Can you work these out from the model? Positions are in its coordinate system, mm. A direction names the side the tool comes from. Give positions to 0.01 mm unless a question says otherwise; leave off trailing zeros. Loops run counter-clockwise (first coordinate to the right, second up) from the corner with the lowest first, then second, coordinate; pieces in that order, holes last. Notation, with made-up numbers: M 38.5,-24.75 L 59.5,-24.75 A31 ccw 59.5,9.25 Z; hole C -8.75,69.5 d7. An arc over 180 degrees is marked long. Answer as a JSON object with one key per item and string values.
Autodesk Fusion 360 part; units mm, degrees
sketch "Sketch1" plane through (0, 0, 0) normal (0, 1, 0) x (1, 0, 0)
  line L0 (32.8, 42.5) -> (-32.8, 42.5)
  line L1 (-32.8, 42.5) -> (-32.8, -42.5)
  line L2 (-32.8, -42.5) -> (32.8, -42.5)
  line L3 (32.8, -42.5) -> (32.8, 42.5)
  line L4 (32.8, 42.5) -> (-32.8, -42.5) construction
  line L5 (-32.8, 42.5) -> (32.8, -42.5) construction
  dimension "d1" = 65.6
  dimension "d2" = 85
extrude "Extrude1" add sketch "Sketch1" along normal blind 20
sketch "Sketch2" plane through (0, 20, 0) normal (0, 1, 0) x (-1, 0, 0)
  line L0 (-32.8, 42.5) -> (-32.8, -42.5)
  line L1 (-32.8, -42.5) -> (32.8, -42.5)
  line L2 (32.8, -42.5) -> (32.8, 42.5)
  line L3 (32.8, 42.5) -> (-32.8, 42.5)
  line L4 (0, 42.5) -> (0, 34.5) construction
  line L5 (0, 34.5) -> (-24.75, 34.5) construction
  line L6 (0, 34.5) -> (24.75, 34.5) construction
  circle A0 centre (24.75, 34.5) radius 3
  circle A1 centre (-24.75, 34.5) radius 3
  dimension "d5" = 8
  dimension "d6" = 24.75
  dimension "d7" = 24.75
  dimension "d8" = 6
  dimension "d9" = 6
extrude "Extrude2" cut sketch "Sketch2" against normal up to surface (20 mm away) contours A0 | A1
ref_plane "WorkPlane1" through (0, 12, 0) normal (0, 1, 0) x (0, 0, 1)
sketch "Sketch3" plane through (0, 12, 0) normal (0, 1, 0) x (1, 0, 0)
  line L0 (20.0157, -34.5) -> (22.3829, -38.6)
  line L1 (22.3829, -38.6) -> (27.1171, -38.6)
  line L2 (27.1171, -38.6) -> (29.4843, -34.5)
  line L3 (29.4843, -34.5) -> (27.1171, -30.4)
  line L4 (27.1171, -30.4) -> (22.3829, -30.4)
  line L5 (22.3829, -30.4) -> (20.0157, -34.5)
  circle A0 centre (24.75, -34.5) radius 3
  line L6 (-20.0157, -34.5) -> (-22.3829, -30.4)
  line L7 (-22.3829, -30.4) -> (-27.1171, -30.4)
  line L8 (-27.1171, -30.4) -> (-29.4843, -34.5)
  line L9 (-29.4843, -34.5) -> (-27.1171, -38.6)
  line L10 (-27.1171, -38.6) -> (-22.3829, -38.6)
  line L11 (-22.3829, -38.6) -> (-20.0157, -34.5)
  circle A1 centre (-24.75, -34.5) radius 3
  point P0 (24.75, -34.5)
  point P1 (-24.75, -34.5)
  dimension "d13" = 4.1
  dimension "d14" = 4.1
extrude "Extrude3" cut sketch "Sketch3" against normal up to surface (12 mm away) contours L0 L1 L2 L3 L4 L5 | A0 | L6 L7 L8 L9 L10 L11 | A1
equation "d6 = ( 49.5 / 2 ) * 1 mm"
equation "d7 = ( 49.5 / 2 ) * 1 mm"
equation "d13 = ( 8.2 / 2 ) * 1 mm"
equation "d14 = ( 8.2 / 2 ) * 1 mm"
1) Suppose I cut it at A-A, the plane y = 2.75. Write out the boundary of the cut face in (x, z).
Answer list:
{"outline": "M -32.8,-42.5 L 32.8,-42.5 L 32.8,42.5 L -32.8,42.5 Z; hole M -29.48,34.5 L -27.12,30.4 L -22.38,30.4 L -20.02,34.5 L -22.38,38.6 L -27.12,38.6 Z; hole M 20.02,34.5 L 22.38,30.4 L 27.12,30.4 L 29.48,34.5 L 27.12,38.6 L 22.38,38.6 Z"}
2) Please list where these lines run through material, in increasing order: line 1 along X through (y, z) = (4.25, 37.5); line 2 along Z through (x, y) = (24.75, 16.5); line 3 along Z through (x, y) = (22, 1.25). Write a range as from..to.
Answer list:
{"line 1": "-32.8..-27.75, -21.75..21.75, 27.75..32.8", "line 2": "-42.5..31.5, 37.5..42.5", "line 3": "-42.5..31.06, 37.94..42.5"}
3) For faces 4 (the flat face through (0, 20, -1)), 5 (the flat face through (25, 6, 38.6)), which set-ups out of +Z, -Z, +X, -X, +Y, -Y let a thin tool reach every point of the face, with its end or its side?
Answer list:
{"face 4": "+Z, -Z, +X, -X, +Y", "face 5": "-Y"}
4) If we mould it in two halves opening along Z, with no side actions, what happens to faces 1 (the flat face through (0, 0, -1)), 2 (the flat face through (0, 10, -42.5)), 3 (the flat face through (28.284, 6.084, 36.579))? For each: +Z half, -Z half, draft (parallel to the pull), parting line (faces both ways), or undercut.
Answer list:
{"face 1": "draft", "face 2": "-Z half", "face 3": "undercut"}
5) Suppose I cut it at B-B, the plane x = -24.75. Write out the boundary of the cut face in (y, z), and give its area (3 significant figures).
Answer list:
{"outline": "M 0,-42.5 L 20,-42.5 L 20,31.5 L 12,31.5 L 12,30.4 L 0,30.4 Z; M 0,38.6 L 12,38.6 L 12,37.5 L 20,37.5 L 20,42.5 L 0,42.5 Z", "area": "1,550 mm^2"}
6) Will this pin go through, and if not, where does the flat tip stop? pin 1 Ø4 at (x, z) = (27, 34.5) entering from -Y.
Answer list:
{"pin 1": "y = 12"}
